Work out the finished part from the listing and answer in its coordinate system (mm). A direction names the side the tool comes from. Round coordinates to 2 decimals unless told otherwise and drop trailing zeros. Use one line per item in the form item = value.
```python
from build123d import *

# Parameters (mm, degrees)
SKETCH1_R           = 28.5
BOSS_EXTRUDE1_DEPTH = 5
CUT_EXTRUDE1_DEPTH  = 6
CIRPATTERN1_COUNT   = 5
SKETCH3_R           = 14
CUT_EXTRUDE2_DEPTH  = 1.5
SKETCH4_R           = 1.5
SKETCH4_R_2         = 6
CUT_EXTRUDE3_DEPTH  = 4.5
SKETCH5_R           = 1.5
CUT_EXTRUDE4_DEPTH  = 6
CIRPATTERN2_COUNT   = 5
FILLET1_R           = 0.5
SKETCH7_R           = 1
BOSS_EXTRUDE2_DEPTH = 20
CIRPATTERN3_COUNT   = 5
SCALE_1_SCALE       = 0.894736842


with BuildPart() as part:
    # Sketch1 → Boss-Extrude1 (new body)
    with BuildSketch(Plane(origin=(0, 0, 0), x_dir=(1, 0, 0), z_dir=(0, 1, 0))):
        Circle(SKETCH1_R)
    extrude(amount=BOSS_EXTRUDE1_DEPTH)

    # Sketch2 → Cut-Extrude1 (cut, through all)
    with BuildSketch(Plane(origin=(0, 5, 0), x_dir=(1, 0, 0), z_dir=(0, 1, 0))):
        with BuildLine():
            Line((10, 26.68801229), (10, 17.68801229))
            ThreePointArc((10, 17.68801229), (0, 16.180315356), (-10, 17.68801229))
            Line((-10, 17.68801229), (-10, 26.68801229))
            ThreePointArc((-10, 26.68801229), (0, 28.5), (10, 26.68801229))
        make_face()
    cut_extrude1 = extrude(amount=-CUT_EXTRUDE1_DEPTH, mode=Mode.SUBTRACT)

    # CirPattern1: Cut-Extrude1 ×5 about axis
    cirpattern1_axis = Axis((0, 0, 0), (0, 1, 0))
    for i in range(1, CIRPATTERN1_COUNT):
        add(cut_extrude1.rotate(cirpattern1_axis, i * 360 / CIRPATTERN1_COUNT), mode=Mode.SUBTRACT)

    # Sketch3 → Cut-Extrude2 (cut)
    with BuildSketch(Plane(origin=(0, 5, 0), x_dir=(1, 0, 0), z_dir=(0, 1, 0))):
        Circle(SKETCH3_R)
    cut_extrude2 = extrude(amount=-CUT_EXTRUDE2_DEPTH, mode=Mode.SUBTRACT)

    # Mirror1: Cut-Extrude2 across plane
    add(cut_extrude2.mirror(Plane.ZX.offset(2.5)), mode=Mode.SUBTRACT)

    # Sketch4 → Cut-Extrude3 (cut, through all)
    with BuildSketch(Plane(origin=(0, 3.5, 0), x_dir=(1, 0, 0), z_dir=(0, 1, 0))):
        with Locations((0, 10.5)):
            Circle(SKETCH4_R)
        with Locations((9.09326674, 5.25)):
            Circle(SKETCH4_R)
        with Locations((9.09326674, -5.25)):
            Circle(SKETCH4_R)
        with Locations((0, -10.5)):
            Circle(SKETCH4_R)
        with Locations((-9.09326674, -5.25)):
            Circle(SKETCH4_R)
        with Locations((-9.09326674, 5.25)):
            Circle(SKETCH4_R)
        Circle(SKETCH4_R_2)
    extrude(amount=-CUT_EXTRUDE3_DEPTH, mode=Mode.SUBTRACT)

    # Sketch5 → Cut-Extrude4 (cut, through all)
    with BuildSketch(Plane(origin=(0, 5, 0), x_dir=(1, 0, 0), z_dir=(0, 1, 0))):
        with Locations((0, -24)):
            Circle(SKETCH5_R)
    cut_extrude4 = extrude(amount=-CUT_EXTRUDE4_DEPTH, mode=Mode.SUBTRACT)

    # CirPattern2: Cut-Extrude4 ×5 about axis
    cirpattern2_axis = Axis((0, 0, 0), (0, 1, 0))
    for i in range(1, CIRPATTERN2_COUNT):
        add(cut_extrude4.rotate(cirpattern2_axis, i * 360 / CIRPATTERN2_COUNT), mode=Mode.SUBTRACT)

    # Fillet1
    fillet1_edges = [part.edges().sort_by_distance(p)[0] for p in [
        (-10, 2.5, -26.68801229),
        (10, 2.5, -26.68801229),
        (10, 2.5, -17.68801229),
        (-10, 2.5, -17.68801229),
        (22.291638052, 2.5, -17.757614507),
        (28.471977939, 2.5, 1.263515819),
        (19.912469293, 2.5, 4.044668769),
        (23.776989981, 2.5, 15.713202966),
        (7.596650093, 2.5, 27.468908012),
        (2.306582823, 2.5, 20.187755062),
        (18.48692271, 2.5, 8.432050017),
        (-7.596650093, 2.5, 27.468908012),
        (-23.776989981, 2.5, 15.713202966),
        (-18.48692271, 2.5, 8.432050017),
        (-2.306582823, 2.5, 20.187755062),
        (-28.471977939, 2.5, 1.263515819),
        (-22.291638052, 2.5, -17.757614507),
        (-13.732129405, 2.5, -14.976461557),
        (-19.912469293, 2.5, 4.044668769),
    ]]
    fillet(fillet1_edges, radius=FILLET1_R)

    # Sketch7 → Boss-Extrude2 (add)
    with BuildSketch(Plane(origin=(-8.090169944, 0, -5.877852523), x_dir=(0.587785252, 0, -0.809016994), z_dir=(0.809016994, 0, 0.587785252))):
        with Locations((-24.059120617, 2.5)):
            Circle(SKETCH7_R)
    boss_extrude2 = extrude(amount=BOSS_EXTRUDE2_DEPTH)

    # CirPattern3: Boss-Extrude2 ×5 about axis
    cirpattern3_axis = Axis((0, 3.5, 0), (0, 1, 0))
    for i in range(1, CIRPATTERN3_COUNT):
        add(boss_extrude2.rotate(cirpattern3_axis, i * 360 / CIRPATTERN3_COUNT))


with BuildPart() as part_1:
    # ｽｹｰﾙ1: scaled about (-0.000351369, 2.5, 0.00037965)
    add(part.part.scale(SCALE_1_SCALE).moved(Location((-3.6986e-05, 0.263157895, 3.9963e-05))))


solid = part_1.part
```
Item 1: Determine the mould class of faces 5 (the cylindrical face through (15.06, 2.47, -20.58)), 6 (the cylindrical face through (-0.291, 2.513, 10.705)), 7 (the cylindrical face through (0.13, 2.16, -20.7)) for opening direction Z: released by +Z, released by -Z, zero draft, split by the parting line, or undercut.
Findings:
face_5 = released by -Z
face_6 = undercut
face_7 = undercut
Item 2: For faces 1 (the cylindrical face through (19.7, 2.8, -6.3)), 2 (the cylindrical face through (0.122, 2.531, -14.477)), 3 (the cylindrical face through (-9.94, 0.92, 7.62)), 4 (the cylindrical face through (-9.94, 4.08, 7.62)), determine the directions among +Z, -Z, +X, -X, +Y, -Y from which every point of the face is accessible in a straight line to the end or side of a thin tool.
Findings:
face_1 = none
face_2 = +Y, -Y
face_3 = -Y
face_4 = +Y
Item 3: The part is cut by section A-A, the plane y = 4. Give the number of separate pieces and of enclosed holes in the cut face, and give its area (3 significant figures).
Findings:
separate_pieces = 1
enclosed_holes = 6
area = 622 mm^2
Item 4: Consider line 1 along Z through (x, y) = (-5.5, 1); line 2 along Z through (x, y) = (2.5, 3.15); line 3 along X through (y, z) = (2.9, -8). Determine where each line is inside the solid, lowest interval first.
Findings:
line_1 = -14.98 to -11.25, 11.25 to 14.21, 22.79 to 24.9
line_2 = -22.14 to -20.91, -14.58 to -4.75, 4.75 to 17.49, 18.66 to 25.38
line_3 = -20.88 to -19.19, -12.85 to 12.85, 19.19 to 20.88
Item 5: Flat-ended cylindrical pins translate along their axes: P1, Ø1.6, axis at x = -20.42, z = 6.64, coming from the +Y side; P2, Ø1, axis at y = 2.5, z = -7, coming from the +X side; P3, Ø3, axis at x = 8.14, z = 4.7, coming from the +Y side; P4, Ø1.5, axis at x = 9.5, z = 4.5, coming from the -Y side. Find the tip coordinate at first contact, or state that the pin passes through.
Findings:
P1 = through
P2 = 21.46
P3 = 3.39
P4 = 1.61
